Verification items for the finished model (mm, model axes). A direction names the side the tool comes from. Give positions to 0.01 mm unless a question says otherwise; leave off trailing zeros. Write each loop counter-clockwise with the first axis right and the second up, starting at its lowest first coordinate (ties: lowest second). Pieces come first, ordered by that corner, then holes. Notation, with made-up numbers: (-28.5, 67) -> (11.5, 67) arc R27 ccw to (11.5, 98) -> close; hole circle Ø8 at (-12, 76). An arc over 180 degrees is marked (long way). Write item = value, one per line.
from build123d import *

# Parameters (mm, degrees)
SKETCH_W        = 55.4
SKETCH_H        = 31.6
PAD_DEPTH       = 75
SKETCH001_W     = 50.4
SKETCH001_H     = 26.6
POCKET_DEPTH    = 72.5
SKETCH002_W     = 1
SKETCH002_H     = 75
PAD001_DEPTH    = 0.8
SKETCH003_W     = 1
SKETCH003_H     = 72.5
PAD002_DEPTH    = 0.8
SKETCH004_W     = 19.1
SKETCH004_H     = 19.09362
POCKET001_DEPTH = 56
FILLET_R        = 1
FILLET001_R     = 1
SKETCH005_W     = 4
SKETCH005_H     = 2.5
POCKET002_DEPTH = 4
FILLET002_R     = 0.75
CHAMFER_SIZE    = 2
FILLET003_R     = 2.5
SKETCH006_W     = 1
SKETCH006_H     = 2.2
POCKET003_DEPTH = 72.5
SKETCH007_W     = 5
SKETCH007_H     = 5
PAD003_DEPTH    = 10
CHAMFER001_SIZE = 4.99
FILLET004_R     = 4.9


with BuildPart() as part:
    # Sketch → Pad (new body)
    with BuildSketch(Plane.XY):
        with Locations((0.5, 0)):
            Rectangle(SKETCH_W, SKETCH_H)
    extrude(amount=PAD_DEPTH)

    # Sketch001 (on Face6 of Pad) → Pocket (cut)
    with BuildSketch(Plane.XY.offset(75)):
        with Locations((0.5, 0)):
            Rectangle(SKETCH001_W, SKETCH001_H)
    extrude(amount=-POCKET_DEPTH, mode=Mode.SUBTRACT)

    # Sketch002 (on Face10 of Pocket) → Pad001 (join)
    with BuildSketch(Plane.YZ.offset(-24.7)):
        with Locations((8.8, 37.5)):
            Rectangle(SKETCH002_W, SKETCH002_H)
        with Locations((6, 37.5)):
            Rectangle(SKETCH002_W, SKETCH002_H)
    extrude(amount=PAD001_DEPTH)

    # Sketch003 (on Face10 of Pad001) → Pad002 (join)
    with BuildSketch(Plane(origin=(25.7, 0, 0), x_dir=(0, -1, 0), z_dir=(-1, 0, 0))):
        with Locations((-8.8, 38.75)):
            Rectangle(SKETCH003_W, SKETCH003_H)
        with Locations((-6, 38.75)):
            Rectangle(SKETCH003_W, SKETCH003_H)
    extrude(amount=PAD002_DEPTH)

    # Sketch004 (on Face3 of Pad002) → Pocket001 (cut)
    with BuildSketch(Plane.YZ.offset(28.2)):
        with Locations((-6.25, 65.45319)):
            Rectangle(SKETCH004_W, SKETCH004_H)
    extrude(amount=-POCKET001_DEPTH, mode=Mode.SUBTRACT)

    # Fillet
    fillet_edges = [part.edges().sort_by_distance(p)[0] for p in [
        (25.7, 11.3, 2.5),
        (0.5, 13.3, 2.5),
        (-24.7, 11.3, 2.5),
    ]]
    fillet(fillet_edges, radius=FILLET_R)

    # Fillet001
    fillet001_edges = [part.edges().sort_by_distance(p)[0] for p in [
        (0.5, -13.3, 2.5),
    ]]
    fillet(fillet001_edges, radius=FILLET001_R)

    # Sketch005 (on Face37 of Fillet001) → Pocket002 (cut)
    with BuildSketch(Plane(origin=(0, 0, 0), x_dir=(1, 0, 0), z_dir=(0, 0, -1))):
        with Locations((16.858666, -0.55)):
            Rectangle(SKETCH005_W, SKETCH005_H)
    extrude(amount=-POCKET002_DEPTH, mode=Mode.SUBTRACT)

    # Fillet002
    fillet002_edges = [part.edges().sort_by_distance(p)[0] for p in [
        (18.858666, 1.8, 1.25),
        (18.858666, -0.7, 1.25),
        (14.858666, -0.7, 1.25),
        (14.858666, 1.8, 1.25),
    ]]
    fillet(fillet002_edges, radius=FILLET002_R)

    # Chamfer
    chamfer_edges = [part.edges().sort_by_distance(p)[0] for p in [
        (16.858666, 1.8, 2.5),
    ]]
    chamfer(chamfer_edges, length=CHAMFER_SIZE)

    # Fillet003
    fillet003_edges = [part.edges().sort_by_distance(p)[0] for p in [
        (-27.2, -15.8, 27.95319),
        (-27.2, 15.8, 37.5),
        (28.2, -15.8, 27.95319),
        (28.2, 15.8, 37.5),
    ]]
    fillet(fillet003_edges, radius=FILLET003_R)

    # Sketch006 (on Face20 of Fillet003) → Pocket003 (cut)
    with BuildSketch(Plane.XY.offset(75)):
        with Locations((-24.4, 7.4)):
            Rectangle(SKETCH006_W, SKETCH006_H)
        with Locations((25.4, 7.4)):
            Rectangle(SKETCH006_W, SKETCH006_H)
    extrude(amount=-POCKET003_DEPTH, mode=Mode.SUBTRACT)

    # Sketch007 (on Face21 of Pocket003) → Pad003 (join)
    with BuildSketch(Plane.XY.offset(55.90638)):
        with Locations((23.2, -10.8)):
            Rectangle(SKETCH007_W, SKETCH007_H)
        with Locations((-22.2, -10.8)):
            Rectangle(SKETCH007_W, SKETCH007_H)
    extrude(amount=-PAD003_DEPTH)

    # Chamfer001
    chamfer001_edges = [part.edges().sort_by_distance(p)[0] for p in [
        (20.7, -10.8, 45.90638),
        (-19.7, -10.8, 45.90638),
    ]]
    chamfer(chamfer001_edges, length=CHAMFER001_SIZE)

    # Fillet004
    fillet004_edges = [part.edges().sort_by_distance(p)[0] for p in [
        (-19.7, -8.3, 53.40138),
        (20.7, -8.3, 53.40138),
    ]]
    fillet(fillet004_edges, radius=FILLET004_R)


solid = part.part
Item 1: Material ranges on line 1 (Y direction, x = 23.5, z = 33.5); line 2 (X direction, y = 10.5, z = 6); line 3 (X direction, y = 6, z = 28), recorded low to high.
Response values:
line_1 = -15.8 to -13.3, 13.3 to 15.8
line_2 = -27.2 to -24.7, 25.7 to 28.2
line_3 = -27.2 to -23.9, 24.9 to 28.2
Item 2: Sectioned sample at D-D on z = 59. Record the cut outline in (x, y).
Response values:
outline = (-27.2, 3.3) -> (-24.7, 3.3) -> (-24.7, 5.5) -> (-23.9, 5.5) -> (-23.9, 6.3) -> (-24.9, 6.3) -> (-24.9, 8.5) -> (-23.9, 8.5) -> (-23.9, 9.3) -> (-24.7, 9.3) -> (-24.7, 13.3) -> (25.7, 13.3) -> (25.7, 9.3) -> (24.9, 9.3) -> (24.9, 8.5) -> (25.9, 8.5) -> (25.9, 6.3) -> (24.9, 6.3) -> (24.9, 5.5) -> (25.7, 5.5) -> (25.7, 3.3) -> (28.2, 3.3) -> (28.2, 13.3) arc R2.5 ccw to (25.7, 15.8) -> (-24.7, 15.8) arc R2.5 ccw to (-27.2, 13.3) -> close
Item 3: Set-up check for faces 5 (the flat face through (-24.7, -4, 32)), 6 (the cylindrical face through (-21.746, -9.217, 51.983)), 7 (the flat face through (27, 3.3, 65)): record each of +Z, -Z, +X, -X, +Y, -Y from which the full face is reachable in a straight line by a thin tool's end or side.
Response values:
face_5 = none
face_6 = +Z
face_7 = +Z, +X, -X, -Y
Item 4: Sectioned sample at B-B on y = -5.5. Record the cut outline in (x, z).
Response values:
outline = (-27.2, 0) -> (28.2, 0) -> (28.2, 55.91) -> (25.7, 55.91) -> (25.7, 3.5) arc R1 cw to (24.7, 2.5) -> (-23.7, 2.5) arc R1 cw to (-24.7, 3.5) -> (-24.7, 55.91) -> (-27.2, 55.91) -> close
Item 5: Mould release check, pull along Y, two halves, no side actions. Record for faces 1 (the flat face through (0, 15.8, 37)), 2 (the flat face through (13.87, 0.56, 1.49)), 3 (the flat face through (0, 0, 0)), 4 (the flat face through (-26, 3.3, 65)): +Y half, -Y half, draft (parallel to the pull), parting line (faces both ways), or undercut.
Response values:
face_1 = +Y half
face_2 = undercut
face_3 = draft
face_4 = -Y half
Item 6: Go/stop test with flat-tipped pins: P1, Ø3, axis at x = 14.5, y = 4, coming from the +Z side; P2, Ø3, axis at x = 11.5, y = 7, coming from the -Z side; P3, Ø3, axis at x = 27, z = 67.5, coming from the -Y side. Record where each tip stops, or that it passes through.
Response values:
P1 = 2.5
P2 = 0
P3 = 3.3
Item 7: Sectioned sample at C-C on x = -8.5. Record the cut outline in (y, z).
Response values:
outline = (-15.8, 0) -> (15.8, 0) -> (15.8, 75) -> (13.3, 75) -> (13.3, 3.5) arc R1 cw to (12.3, 2.5) -> (-12.3, 2.5) arc R1 cw to (-13.3, 3.5) -> (-13.3, 55.91) -> (-15.8, 55.91) -> close
